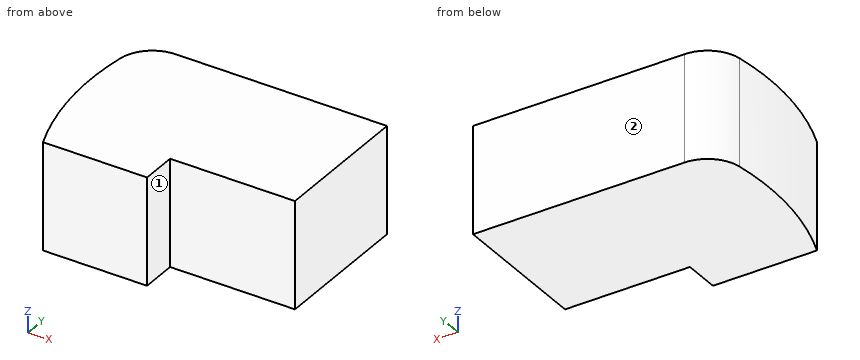
from build123d import *

# Parameters (mm, degrees)
F1_DEPTH = 38.1
F2_R     = 12.7


with BuildPart() as f1:
    # F0 (on Top) → F1 (new body)
    with BuildSketch(Plane.XY):
        with BuildLine():
            ThreePointArc((3.226223, 63.5), (0.220256, 31.413637), (7.414279, 0))
            Line((7.414279, 0), (44.45, 0))
            Line((44.45, 0), (44.45, 12.7))
            Line((44.45, 12.7), (88.9, 12.7))
            Line((88.9, 12.7), (88.9, 63.5))
            Line((88.9, 63.5), (3.226223, 63.5))
        make_face()
    extrude(amount=F1_DEPTH)

    # F2
    f2_edges = [f1.edges().sort_by_distance(p)[0] for p in [
        (3.226223, 63.5, 19.05),
    ]]
    fillet(f2_edges, radius=F2_R)


solid = f1.part
Verification items for the finished model (mm, model axes). Face numbers are marked on the shaded views. A direction names the side the tool comes from. Coordinates: 2 decimals unless noted, no trailing zeros. Order: outer loops, then holes, each group sorted by start corner. A loop starts at its lowest first (then second) coordinate and runs counter-clockwise, first axis right, second up.
Item 1: Material ranges on L1, parallel to Y at x = 70, z = 29.5; L2, parallel to X at y = 39, z = 31.5; L3, parallel to X at y = 26.5, z = 31.5, recorded low to high.
Filled in:
L1: y = 12.7 to 63.5
L2: x = 0 to 88.9
L3: x = 0.66 to 88.9
Item 2: Section check C-C, the plane y = 4. Enter the section's corners in (x, z), then the cut area to 3 significant figures.
Filled in:
outline: (5.89, 0) - (44.45, 0) - (44.45, 38.1) - (5.89, 38.1) - close
area: 1,470 mm2
Item 3: Section check B-B, the plane x = 69.5. Enter the section's corners in (y, z), then the cut area to 3 significant figures.
Filled in:
outline: (12.7, 0) - (63.5, 0) - (63.5, 38.1) - (12.7, 38.1) - close
area: 1,940 mm2
Item 4: Depth check by flat-ended pin: pin 1 (1.5 mm diameter, centred on y = 40, z = 24, fed in from -X); pin 2 (4 mm diameter, centred on y = 9, z = 16.5, fed in from +X); pin 3 (4 mm diameter, centred on x = 18, y = 49, fed in from -Z). Enter the tip coordinate at first touch or a pass-through.
Filled in:
pin 1: stops at x = 0.01
pin 2: stops at x = 44.45
pin 3: stops at z = 0
Item 5: Access from +Z, -Z, +X, -X, +Y, -Y to the whole of each face (thin tool, end or side, straight path). Record for the marked faces 1 and 2.
Filled in:
face 1: +Z, -Z, +X, -Y
face 2: +Z, -Z, +X, -X, +Y
Item 6: Section check A-A, the plane z = 17. Enter the section's corners in (x, y), then the cut area to 3 significant figures.
Filled in:
outline: (1.04, 52.61) arc R101.6 ccw to (7.41, 0) - (44.45, 0) - (44.45, 12.7) - (88.9, 12.7) - (88.9, 63.5) - (13.61, 63.5) arc R12.7 ccw to start
area: 4,940 mm2
